from build123d import *

# Parameters (mm, degrees)
SKETCH2_R           = 10
BOSS_EXTRUDE5_DEPTH = 20
CUT_EXTRUDE1_DEPTH  = 20


with BuildPart() as part:
    # Sketch2 → Boss-Extrude5 (new body)
    with BuildSketch(Plane(origin=(0, 0, 0), x_dir=(0, 0, -1), z_dir=(1, 0, 0))):
        Circle(SKETCH2_R)
    extrude(amount=BOSS_EXTRUDE5_DEPTH)

    # Sketch5 → Cut-Extrude1 (cut)
    with BuildSketch(Plane(origin=(20, 0, 0), x_dir=(0, 0, -1), z_dir=(1, 0, 0))):
        Polygon((8, 0), (5.656854249, 5.656854249), (0, 8), (-5.656854249, 5.656854249), (-8, 0), (-5.656854249, -5.656854249), (0, -8), (5.656854249, -5.656854249), align=None)
    extrude(amount=-CUT_EXTRUDE1_DEPTH, mode=Mode.SUBTRACT)


solid = part.part
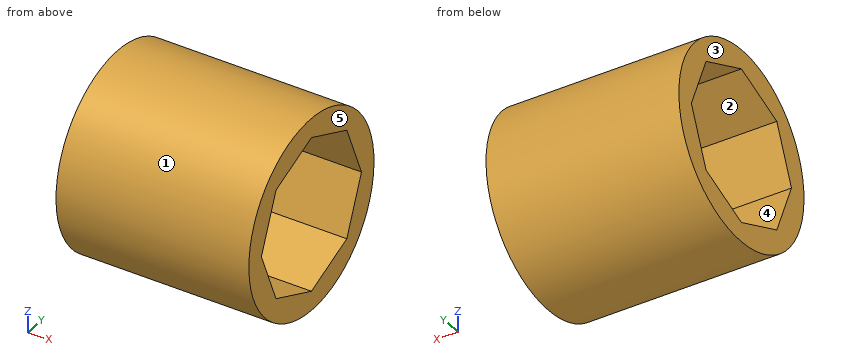
Design review of the part built by this model. Coordinates are the model's own, in mm. Face numbers are marked on the shaded views. A direction names the side the tool comes from. Coordinates: 2 decimals unless noted, no trailing zeros. Loops run counter-clockwise (first coordinate to the right, second up) from the corner with the lowest first, then second, coordinate; pieces in that order, holes last. Notation, with made-up numbers: (34.25, 75) - (80.25, 75) arc R21 cw to (80.25, 103) - close; hole circle Ø4 at (-37, 71.5). An arc over 180 degrees is marked (long way). Use CSV: the item, a comma, the result in double quotes. Start each with the question number.
1. Mouldability with a two-part tool opening along Z and no side actions: class the marked faces 1, 2 and 3 as released by +Z, released by -Z, zero draft, split by the parting line, or undercut.
2. Add section A-A on y = -0.5. Give the boundary of the cut face in (x, z).
3. Add section B-B on z = 5. Give the boundary of the cut face in (x, y).
4. To check wall thickness, follow probe 1 along Y at (x, z) = (12.75, 4.5); probe 2 along Y at (x, z) = (10.75, 4.75); probe 3 along Z at (x, y) = (18.5, 5.25). State the ranges of each line that lie inside material, in increasing order.
5. Add section C-C on x = 17.75. Give the boundary of the cut face in (y, z).
6. Add section D-D on y = -8.5. Give the boundary of the cut face in (x, z), plus the area to 3 significant figures.
7. Clearance check with flat-ended pins moving along their axes: pin 1 (6 mm diameter, centred on x = 17, z = 7.5, fed in from +Y); pin 2 (4 mm diameter, centred on x = 11, z = 5, fed in from -Y); pin 3 (3 mm diameter, centred on x = 9, z = -7.5, fed in from +Y). State where each tip first meets the part, or that it passes through.
8. For the marked faces 4 and 5, list the 3-axis set-ups (+Z, -Z, +X, -X, +Y, -Y) from which the entire face can be reached by the end or side of a thin tool; tool diameter is ignored.
Resolved:
1,face 1,"split by the parting line"
1,face 2,"undercut"
1,face 3,"zero draft"
2,outline,"(0, -9.99) - (20, -9.99) - (20, -7.79) - (0, -7.79) - close; (0, 7.79) - (20, 7.79) - (20, 9.99) - (0, 9.99) - close"
3,outline,"(0, -8.66) - (20, -8.66) - (20, -5.93) - (0, -5.93) - close; (0, 5.93) - (20, 5.93) - (20, 8.66) - (0, 8.66) - close"
4,probe 1,"-8.93 to -6.14, 6.14 to 8.93"
4,probe 2,"-8.8 to -6.03, 6.03 to 8.8"
4,probe 3,"-8.51 to -5.83, 5.83 to 8.51"
5,outline,"circle Ø20 at (0, 0); hole (-8, 0) - (-5.66, -5.66) - (0, -8) - (5.66, -5.66) - (8, 0) - (5.66, 5.66) - (0, 8) - (-5.66, 5.66) - close"
6,outline,"(0, -5.27) - (20, -5.27) - (20, 5.27) - (0, 5.27) - close"
6,area,"211 mm2"
7,pin 1,"y = 8.93"
7,pin 2,"y = -9.54"
7,pin 3,"y = 8"
8,face 4,"+X, -X"
8,face 5,"+Z, -Z, +X, +Y, -Y"
